from build123d import *

# Parameters (mm, degrees)
F1_DEPTH = 6.75
F2_R     = 8
F3_R     = 1.5


with BuildPart() as f1:
    # F0 (on Front) → F1 (new body)
    with BuildSketch(Plane.XZ):
        Polygon((-90.6164456464, 33.1331632659), (-102.6164456464, 33.1331632659), (-102.6164456464, 26.3831632659), (-102.6164456464, -25.1168367341), (-110.6164456464, -25.1168367341), (-110.6164456464, -31.8668367341), (-102.6164456464, -31.8668367341), (-90.6164456464, -31.8668367341), (-90.6164456464, -25.1168367341), (-90.6164456464, 26.3831632659), (-82.6164456464, 26.3831632659), (-82.6164456464, 33.1331632659), align=None)
    extrude(amount=F1_DEPTH)

    # F2
    f2_edges = [f1.edges().sort_by_distance(p)[0] for p in [
        (-102.616446, -3.375, 33.133163),
        (-90.616446, -3.375, -31.866837),
    ]]
    fillet(f2_edges, radius=F2_R)

    # F3
    f3_edges = [f1.edges().sort_by_distance(p)[0] for p in [
        (-102.616446, 0, 0.008163),
        (-106.616446, 0, -25.116837),
        (-102.616446, -6.75, 0.008163),
        (-106.616446, -6.75, -25.116837),
        (-102.616446, -3.375, -25.116837),
        (-104.616446, -6.75, -31.866837),
        (-104.616446, 0, -31.866837),
        (-90.616446, -3.375, 26.383163),
        (-100.2733, 0, 30.790018),
        (-88.616446, 0, 33.133163),
        (-86.616446, 0, 26.383163),
        (-92.959591, 0, -29.523691),
        (-90.616446, 0, 1.258163),
        (-100.2733, -6.75, 30.790018),
        (-88.616446, -6.75, 33.133163),
        (-86.616446, -6.75, 26.383163),
        (-92.959591, -6.75, -29.523691),
        (-90.616446, -6.75, 1.258163),
    ]]
    fillet(f3_edges, radius=F3_R)


solid = f1.part
Can you work these out from the model? Positions are in its coordinate system, mm. A direction names the side the tool comes from. Round coordinates to 2 decimals unless told otherwise and drop trailing zeros. Write each loop counter-clockwise with the first axis right and the second up, starting at its lowest first coordinate (ties: lowest second). Pieces come first, ordered by that corner, then holes. Notation, with made-up numbers: M 80,-34.5 L 110,-34.5 A8 cw 110,-21.5 Z; hole C 23.25,61 d3. An arc over 180 degrees is marked long. Use CSV: the item, a comma, the result in double quotes.
(1) I need wall thicknesses on line 1 along Z through (x, y) = (-107.25, -2); line 2 along X through (y, z) = (-5.25, -15); line 3 along Z through (x, y) = (-98, -1). Which ranges of each line are inside material? Lowest first, please.
Check values:
line 1,"-31.87 to -25.12"
line 2,"-102.62 to -90.62"
line 3,"-31.76 to 32.29"
(2) Imagine slicing it at B-B (z = 8). Write out the boundary of the cut face in (x, y).
Check values:
outline,"M -102.62,-5.25 A1.5 ccw -101.12,-6.75 L -92.12,-6.75 A1.5 ccw -90.62,-5.25 L -90.62,-1.5 A1.5 ccw -92.12,0 L -101.12,0 A1.5 ccw -102.62,-1.5 Z"
(3) On a 3-axis mill with a long thin cutter (end or side, diameter ignored), from which of +Z, -Z, +X, -X, +Y, -Y can I reach the whole of each face in a straight line? I mean faces 1 (the cylindrical face through (-85.82, -0.43, 26.83)), 2 (the flat face through (-90.616, -3, 0)), 3 (the flat face through (-102.616, -3, 1)), 4 (the cylindrical face through (-102.19, -6.3, 0.42)), 5 (the cylindrical face through (-107.412, -0.428, -25.568)). Say none if no direction works.
Check values:
face 1,"-Z, +X, +Y"
face 2,"-Z, +X, +Y, -Y"
face 3,"+Z, -X, +Y, -Y"
face 4,"+Z, -X, -Y"
face 5,"+Z, -X, +Y"
(4) I'm going to push flat-ended pins straight in: pin 1 (3 mm diameter, centred on y = -4.5, z = 2.5, fed in from +X); pin 2 (4 mm diameter, centred on x = -86, y = -2.5, fed in from -Z); pin 3 (8 mm diameter, centred on x = -88.5, z = 18, fed in from -Y); pin 4 (5 mm diameter, centred on x = -88, z = -13.5, fed in from -Y). Where does each tip first touch, or does it pass through?
Check values:
pin 1,"x = -90.62"
pin 2,"z = 26.38"
pin 3,"y = -6.75"
pin 4,"through"
(5) Imagine slicing it at A-A (y = -4.5). Write out the boundary of the cut face in (x, z).
Check values:
outline,"M -110.62,-31.87 L -98.62,-31.87 A8 ccw -90.62,-23.87 L -90.62,24.88 A1.5 cw -89.12,26.38 L -82.62,26.38 L -82.62,33.13 L -94.62,33.13 A8 ccw -102.62,25.13 L -102.62,-23.62 A1.5 cw -104.12,-25.12 L -110.62,-25.12 Z"
(6) Imagine slicing it at C-C (x = -106.25). Write out the boundary of the cut face in (y, z), plus the area to 3 significant figures.
Check values:
outline,"M -6.75,-30.37 A1.5 ccw -5.25,-31.87 L -1.5,-31.87 A1.5 ccw 0,-30.37 L 0,-26.62 A1.5 ccw -1.5,-25.12 L -5.25,-25.12 A1.5 ccw -6.75,-26.62 Z"
area,"43.6 mm^2"
